Study the drawing (mm; zero at the part's minimum x, y, z) and answer. A direction names the side the tool comes from. Coordinates: 2 decimals unless noted, no trailing zeros. Loops run counter-clockwise (first coordinate to the right, second up) from the corner with the lowest first, then second, coordinate; pieces in that order, holes last. Notation, with made-up numbers: (10.5, -13) - (19.5, -13) arc R29 ccw to (19.5, 25) - close; hole circle Ø9 at (28, 25). An arc over 180 degrees is marked (long way). Use one line per item in the form item = value.
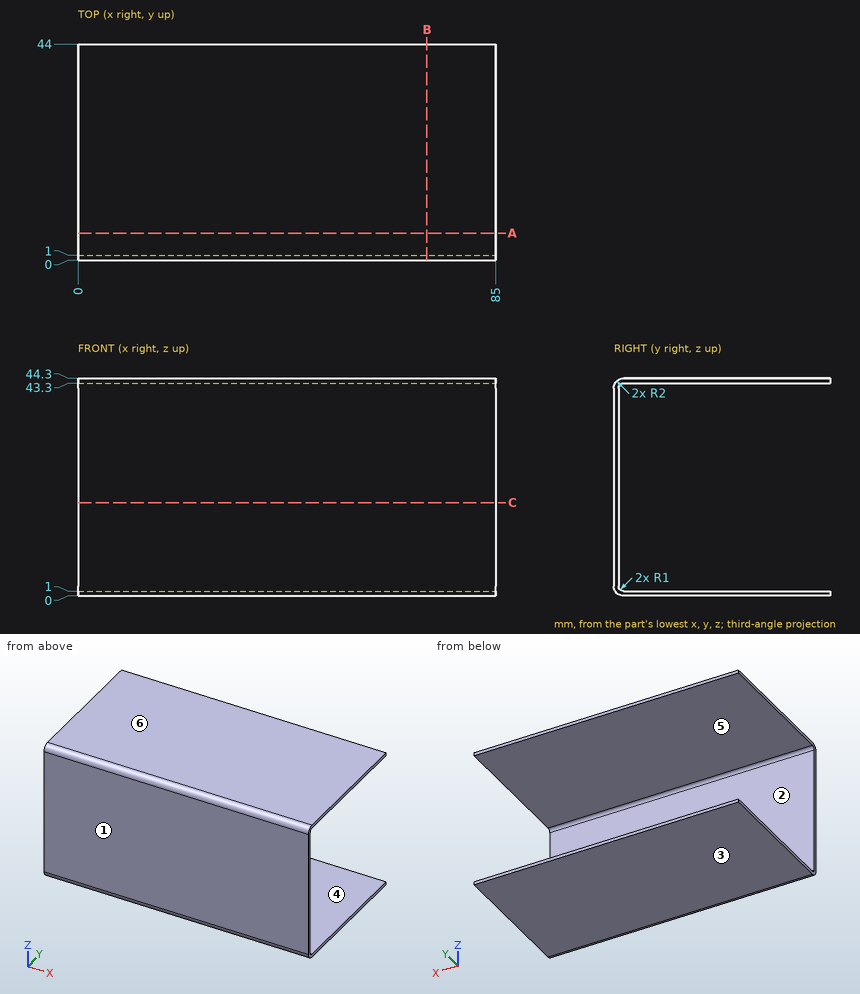
Item 1: The part is cut by section A-A on y = 5.5. Give the vertices of the cut face in (x, z), plus the area to 3 significant figures.
Results below:
outline = (0, 0) - (85, 0) - (85, 1) - (0, 1) - close; (0, 43.3) - (85, 43.3) - (85, 44.3) - (0, 44.3) - close
area = 170 mm²
Item 2: Find the intervals of material crossed by L1, parallel to Z at x = 30, y = 3; L2, parallel to Y at x = 15, z = 17.5, in increasing order.
Results below:
L1 = 0 to 1, 43.3 to 44.3
L2 = 0 to 1
Item 3: Which of the six approach directions +Z, -Z, +X, -X, +Y, -Y give full straight-line access (tool end or side, diameter ignored) to the marked faces 1 and 2?
Results below:
face_1 = +Z, -Z, +X, -X, -Y
face_2 = +X, -X, +Y
Item 4: The part is cut by section C-C on z = 19. Give the vertices of the cut face in (x, y), plus the area to 3 significant figures.
Results below:
outline = (0, 0) - (85, 0) - (85, 1) - (0, 1) - close
area = 85.0 mm²
Item 5: The part is cut by section B-B on x = 71. Give the vertices of the cut face in (y, z), plus the area to 3 significant figures.
Results below:
outline = (0, 2) arc R2 ccw to (2, 0) - (44, 0) - (44, 1) - (2, 1) arc R1 cw to (1, 2) - (1, 42.3) arc R1 cw to (2, 43.3) - (44, 43.3) - (44, 44.3) - (2, 44.3) arc R2 ccw to (0, 42.3) - close
area = 129 mm²
Item 6: Each of these flat-tipped pins is pushed along its axis until it touches: P1, Ø5, axis at x = 75, y = 4.5, coming from the -Z side; P2, Ø10, axis at x = 27, z = 18.5, coming from the +Y side. Where does it stop, or does it pass through?
Results below:
P1 = 0
P2 = 1
Item 7: For a pull along Z with two mould halves and no side action, classify the marked faces 3, 4, 5 and 6 as +Z half, -Z half, draft (parallel to the pull), parting line (faces both ways), or undercut.
Results below:
face_3 = -Z half
face_4 = undercut
face_5 = undercut
face_6 = +Z half
